Part model, mm, in its own coordinate system. A direction names the side the tool comes from. Coordinates: 2 decimals unless noted, no trailing zeros. Loops run counter-clockwise (first coordinate to the right, second up) from the corner with the lowest first, then second, coordinate; pieces in that order, holes last. Notation, with made-up numbers: (83.25, 34.25) - (98.25, 34.25) arc R20 ccw to (98.25, 39.25) - close; hole circle Ø5 at (-34.5, 80). An arc over 180 degrees is marked (long way). Use a Markdown table: item, result. Add a question column.
1. 3-axis set-ups, long thin cutter, end or side, ignore diameter. For faces 1 (the flat face through (0, 0, 4)), 2 (the flat face through (102.5, 0, -15)), 3 (the flat face through (5, 16, 12)), 4 (the cylindrical face through (5, 0, -16)): which of +Z, -Z, +X, -X, +Y, -Y reach the whole face in a straight line?
2. Drop flat-ended pins along their axis: pin 1 (1.5 mm diameter, centred on y = -0.5, z = 15.5, fed in from +X); pin 2 (2.5 mm diameter, centred on y = 0, z = -15.5, fed in from +X); pin 3 (5 mm diameter, centred on x = 18, z = -8.5, fed in from -Y); pin 4 (3.5 mm diameter, centred on y = 0, z = 15, fed in from -X). Give the stop position or say it passes through.
3. Pull direction Z, two halves, no side cores. Call faces 5 (the flat face through (5, 0, 25)), 6 (the flat face through (102.5, 0, 15)), 7 (the flat face through (5, -16, 12)): pulls with the +Z half, pulls with the -Z half, needs draft (parallel to the pull), parting line crosses it, or undercut.
4. Band-saw the part on C-C, the plane x = 53.5. Give the cut face in (y, z).
5. Band-saw the part on D-D, the plane y = 7. Give the cut face in (x, z).
6. Band-saw the part on A-A, the plane y = 0. Give the cut face in (x, z).
7. Band-saw the part on B-B, the plane z = 15. Give the cut face in (x, y).
8. Wall check: probe 1 along Y at (x, z) = (106.25, 0); probe 2 along Y at (x, z) = (111, 0); probe 3 along X at (y, z) = (10.5, 18). Give the ranges that are in metal, low to high. Write a range as [from, to].
from build123d import *

# Parameters (mm, degrees)
SKETCH_2_R           = 18
EXTRUDE_1_DEPTH      = 110.5
SKETCH_3_R           = 11
EXTRUDE_2_DEPTH      = 2
SKETCH_4_R           = 4
EXTRUDE_3_DEPTH      = 15
SKETCH_5_R           = 16
SKETCH_5_W           = 25
SKETCH_5_H           = 32
EXTRUDE_4_DEPTH      = 19
CUT_EXTRUDE_START    = -17
SKETCH_6_R           = 4
CUT_EXTRUDE_2_DEPTH  = 17
SKETCH_8_R           = 1.5
CUT_EXTRUDE_3_DEPTH  = 8
SKETCH_9_W           = 7
SKETCH_9_H           = 53.664009665
CUT_EXTRUDE_4_DEPTH  = 121.15510809
SKETCH_10_W          = 2
SKETCH_10_H          = 52.133274579
CUT_EXTRUDE_6_DEPTH  = 121.15510809
EXTRUDE_START        = -20
EXTRUDE_5_DEPTH      = 20
SKETCH_12_R          = 18
SKETCH_12_R_2        = 16
CUT_EXTRUDE_7_DEPTH  = 20
SKETCH_13_W          = 25
SKETCH_13_H          = 32
EXTRUDE_6_DEPTH      = 20
SKETCH_14_W          = 10
SKETCH_14_H          = 32
CUT_EXTRUDE_8_DEPTH  = 122.775408026
SKETCH_15_R          = 18
CUT_EXTRUDE_10_DEPTH = 10
SKETCH_16_R          = 16
EXTRUDE_7_DEPTH      = 10
SKETCH_17_W          = 25
SKETCH_17_H          = 32
EXTRUDE_8_DEPTH      = 10


with BuildPart() as part:
    # Sketch 2 → Extrude 1 (new body)
    with BuildSketch(Plane(origin=(0, 0, 0), x_dir=(0, 0, -1), z_dir=(1, 0, 0))):
        Circle(SKETCH_2_R)
    extrude(amount=EXTRUDE_1_DEPTH)

    # Sketch 3 → Extrude 2 (add)
    with BuildSketch(Plane(origin=(110.5, 0, 0), x_dir=(0, 0, -1), z_dir=(1, 0, 0))):
        Circle(SKETCH_3_R)
    extrude(amount=EXTRUDE_2_DEPTH)

    # Sketch 4 → Extrude 3 (add)
    with BuildSketch(Plane(origin=(112.5, 0, 0), x_dir=(0, 0, -1), z_dir=(1, 0, 0))):
        Circle(SKETCH_4_R)
    extrude(amount=EXTRUDE_3_DEPTH)

    # Sketch 5 → Extrude 4 (add)
    with BuildSketch(Plane.ZY):
        Circle(SKETCH_5_R)
        with Locations((12.5, 0)):
            Rectangle(SKETCH_5_W, SKETCH_5_H)
    extrude(amount=EXTRUDE_4_DEPTH)

    # Sketch 6 → Cut-Extrude 2 (cut)
    with BuildSketch(Plane(origin=(127.5, 0, 0), x_dir=(0, 0, -1), z_dir=(1, 0, 0)).offset(CUT_EXTRUDE_START)):
        Circle(SKETCH_6_R)
    extrude(amount=CUT_EXTRUDE_2_DEPTH, mode=Mode.SUBTRACT)

    # Sketch 8 → Cut-Extrude 3 (cut)
    with BuildSketch(Plane(origin=(110.5, 0, 0), x_dir=(0, 0, -1), z_dir=(1, 0, 0))):
        with Locations((0, 15)):
            Circle(SKETCH_8_R)
        with Locations((15, 0)):
            Circle(SKETCH_8_R)
        with Locations((0, -15)):
            Circle(SKETCH_8_R)
        with Locations((-15, 0)):
            Circle(SKETCH_8_R)
    extrude(amount=-CUT_EXTRUDE_3_DEPTH, mode=Mode.SUBTRACT)

    # Sketch 9 → Cut-Extrude 4 (cut, through all)
    with BuildSketch(Plane.XZ.offset(16)):
        with Locations((-15.5, -1.832004833)):
            Rectangle(SKETCH_9_W, SKETCH_9_H)
    extrude(amount=-CUT_EXTRUDE_4_DEPTH, mode=Mode.SUBTRACT)

    # Sketch 10 → Cut-Extrude 6 (cut, through all)
    with BuildSketch(Plane.XZ.offset(16)):
        with Locations((-11, -1.06663729)):
            Rectangle(SKETCH_10_W, SKETCH_10_H)
    extrude(amount=-CUT_EXTRUDE_6_DEPTH, mode=Mode.SUBTRACT)

    # Sketch 11 → Extrude 5 (add)
    with BuildSketch(Plane.ZY.offset(10).offset(EXTRUDE_START)):
        with BuildLine():
            Line((25, -16), (25, 16))
            Line((25, 16), (0, 16))
            ThreePointArc((0, 16), (11.313708499, 11.313708499), (16, 0))
            ThreePointArc((16, 0), (11.313708499, -11.313708499), (0, -16))
            Line((0, -16), (25, -16))
        make_face()
        with BuildLine():
            Line((0, 16), (0, -16))
            ThreePointArc((0, -16), (-16, 0), (0, 16))
        make_face()
        with BuildLine():
            ThreePointArc((16, 0), (11.313708499, 11.313708499), (0, 16))
            Line((0, 16), (0, -16))
            ThreePointArc((0, -16), (11.313708499, -11.313708499), (16, 0))
        make_face()
        with BuildLine():
            Line((0, -16), (0, 16))
            ThreePointArc((0, 16), (-16, 0), (0, -16))
        make_face()
    extrude(amount=EXTRUDE_5_DEPTH)

    # Sketch 12 → Cut-Extrude 7 (cut)
    with BuildSketch(Plane.ZY):
        with Locations(Location((0, 0, 0), (0, 0, 62.733955549))):
            Circle(SKETCH_12_R)
        Circle(SKETCH_12_R_2, mode=Mode.SUBTRACT)
    extrude(amount=CUT_EXTRUDE_7_DEPTH, mode=Mode.SUBTRACT)

    # Sketch 13 → Extrude 6 (add)
    with BuildSketch(Plane.ZY.offset(10)):
        with Locations((12.5, 0)):
            Rectangle(SKETCH_13_W, SKETCH_13_H)
    extrude(amount=-EXTRUDE_6_DEPTH)

    # Sketch 14 → Cut-Extrude 8 (cut, through all)
    with BuildSketch(Plane.XY.offset(25)):
        with Locations((-5, 0)):
            Rectangle(SKETCH_14_W, SKETCH_14_H)
    extrude(amount=-CUT_EXTRUDE_8_DEPTH, mode=Mode.SUBTRACT)

    # Sketch 15 → Cut-Extrude 10 (cut)
    with BuildSketch(Plane.ZY):
        Circle(SKETCH_15_R)
    extrude(amount=-CUT_EXTRUDE_10_DEPTH, mode=Mode.SUBTRACT)


with BuildPart() as cut_extrude_10_piece_1:
    # of the separate pieces the step leaves, piece 1, a body of its own (cut_extrude_10_pieces)
    add(part.part.solids().sort_by_distance((10, 0, -18))[0])

    # Sketch 16 → Extrude 7 (add)
    with BuildSketch(Plane.ZY.offset(-10)):
        Circle(SKETCH_16_R)
    extrude(amount=EXTRUDE_7_DEPTH)



with BuildPart() as cut_extrude_10_piece_2:
    # of the separate pieces the step leaves, piece 2, a body of its own (cut_extrude_10_pieces)
    add(part.part.solids().sort_by_distance((10, 16, 25))[0])


with BuildPart() as cut_extrude_10_piece_1_1:
    add(cut_extrude_10_piece_1.part)

    add(cut_extrude_10_piece_2.part)  # Extrude 8 merges Cut-Extrude 10 piece 2
    # Sketch 17 → Extrude 8 (add)
    with BuildSketch(Plane.ZY):
        with Locations((12.5, 0)):
            Rectangle(SKETCH_17_W, SKETCH_17_H)
    extrude(amount=-EXTRUDE_8_DEPTH)


solid = cut_extrude_10_piece_1_1.part
Geometry check:
| question | item | result |
|---|---|---|
| 1 | face 1 | +Z, -Z, -X, +Y, -Y |
| 1 | face 2 | +X |
| 1 | face 3 | +Z, -Z, -X, +Y |
| 1 | face 4 | -Z, -X |
| 2 | pin 1 | stops at x = 102.5 |
| 2 | pin 2 | stops at x = 110.5 |
| 2 | pin 3 | stops at y = -16.97 |
| 2 | pin 4 | stops at x = 0 |
| 3 | face 5 | pulls with the +Z half |
| 3 | face 6 | undercut |
| 3 | face 7 | needs draft |
| 4 | outline | circle Ø36 at (0, 0) |
| 5 | outline | (0, -14.39) - (10, -14.39) - (10, -16.58) - (110.5, -16.58) - (110.5, -8.49) - (112.5, -8.49) - (112.5, 8.49) - (110.5, 8.49) - (110.5, 16.58) - (10, 16.58) - (10, 25) - (0, 25) - close |
| 6 | outline | (0, -16) - (10, -16) - (10, -18) - (110.5, -18) - (110.5, -16.5) - (102.5, -16.5) - (102.5, -13.5) - (110.5, -13.5) - (110.5, -11) - (112.5, -11) - (112.5, -4) - (110.5, -4) - (110.5, 4) - (112.5, 4) - (112.5, 11) - (110.5, 11) - (110.5, 13.5) - (102.5, 13.5) - (102.5, 16.5) - (110.5, 16.5) - (110.5, 18) - (10, 18) - (10, 25) - (0, 25) - close |
| 7 | outline | (0, -16) - (10, -16) - (10, -9.95) - (110.5, -9.95) - (110.5, -1.5) - (102.5, -1.5) - (102.5, 1.5) - (110.5, 1.5) - (110.5, 9.95) - (10, 9.95) - (10, 16) - (0, 16) - close |
| 8 | probe 1 | y = [-18, -16.5], [-13.5, 13.5], [16.5, 18] |
| 8 | probe 2 | y = [-11, -4], [4, 11] |
| 8 | probe 3 | x = [0, 10] |
